Geometry check sheet. Reference: the model listing, model coordinates, mm. Face numbers are marked on the shaded views. A direction names the side the tool comes from. Coordinates: 2 decimals unless noted, no trailing zeros. Loops run counter-clockwise (first coordinate to the right, second up) from the corner with the lowest first, then second, coordinate; pieces in that order, holes last.
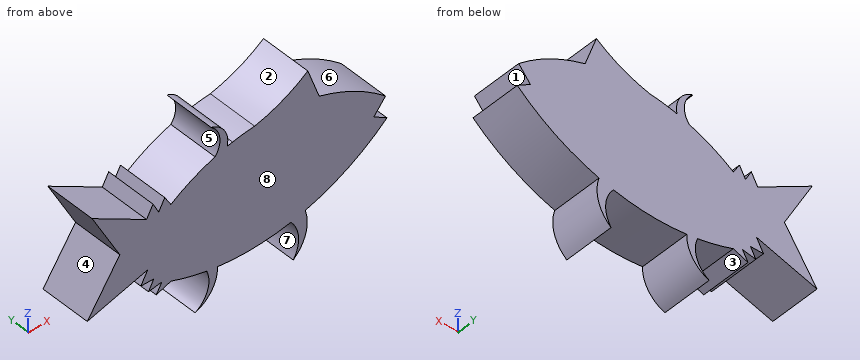
from build123d import *

# Parameters (mm, degrees)
F0_R     = 2.7728075116
F1_DEPTH = 25.4


with BuildPart() as f1:
    # F0 (on Front) → F1 (new body)
    with BuildSketch(Plane.XZ):
        with BuildLine():
            Line((-46.2063811719, 22.3736166954), (-73.4438300133, 37.6946814358))
            Line((-73.4438300133, 37.6946814358), (-59.5819167793, 12.4027663842))
            Line((-59.5819167793, 12.4027663842), (-75.8757442236, -11.4300008863))
            Line((-75.8757442236, -11.4300008863), (-45.6002619536, -2.5907051222))
            ThreePointArc((-45.6002619536, -2.5907051222), (-44.4025685397, -5.830070686), (-42.5679523522, -8.7561845276))
            ThreePointArc((-42.5679523522, -8.7561845276), (-40.7090131833, -10.7730955419), (-38.5467331667, -12.4607359072))
            ThreePointArc((-38.5467331667, -12.4607359072), (-37.5331692858, -13.0762341628), (-36.4787243307, -13.6187244207))
            ThreePointArc((-36.4787243307, -13.6187244207), (-35.218191008, -14.1097204461), (-33.9515178698, -14.5846525628))
            ThreePointArc((-33.9515178698, -14.5846525628), (-25.1236949217, -17.4009018565), (-16.0843420418, -19.4385027989))
            ThreePointArc((-16.0843420418, -19.4385027989), (-13.3899281297, -19.8880494602), (-10.6848629515, -20.2682874284))
            ThreePointArc((-10.6848629515, -20.2682874284), (7.7554033628, -21.0061419822), (26.0458368353, -18.5468952528))
            ThreePointArc((26.0458368353, -18.5468952528), (29.6524190677, -17.6722711402), (33.2263105994, -16.6724201227))
            ThreePointArc((33.2263105994, -16.6724201227), (54.9868951593, -7.4326700378), (74.1704591011, 6.3835123767))
            Line((74.1704591011, 6.3835123767), (67.6072314382, 10.4572335258))
            Line((67.6072314382, 10.4572335258), (73.4438300133, 17.5097864121))
            ThreePointArc((73.4438300133, 17.5097864121), (57.8267715443, 28.3623597624), (40.2292326492, 35.5732881621))
            ThreePointArc((40.2292326492, 35.5732881621), (24.2028822223, 38.5907293118), (7.8949533391, 38.5729912726))
            ThreePointArc((7.8949533391, 38.5729912726), (2.4157752889, 37.4790688574), (-3.1311035908, 36.8081045884))
            ThreePointArc((-3.1311035908, 36.8081045884), (-4.4740862067, 36.4927174845), (-5.8119143408, 36.1561358224))
            ThreePointArc((-5.8119143408, 36.1561358224), (-8.868524213, 35.3017374622), (-11.8920366653, 34.3367333588))
            ThreePointArc((-11.8920366653, 34.3367333588), (-23.3557486049, 29.5105094754), (-34.0166780636, 23.1031924486))
            Line((-34.0166780636, 23.1031924486), (-40.1115296178, 22.738404572))
            Line((-40.1115296178, 22.738404572), (-46.2063811719, 22.3736166954))
        make_face()
        with Locations((53.9885126054, 20.9144670516)):
            Circle(F0_R, mode=Mode.SUBTRACT)
        with BuildLine():
            ThreePointArc((34.5331951976, 51.0702133179), (21.8513167895, 43.4632987988), (7.8949533391, 38.5729912726))
            ThreePointArc((7.8949533391, 38.5729912726), (24.2028822223, 38.5907293118), (40.2292326492, 35.5732881621))
            Line((40.2292326492, 35.5732881621), (34.5331951976, 51.0702133179))
        make_face()
        with BuildLine():
            ThreePointArc((33.2263105994, -16.6724201227), (29.6524190677, -17.6722711402), (26.0458368353, -18.5468952528))
            ThreePointArc((26.0458368353, -18.5468952528), (29.9013197265, -27.9179314628), (27.237445116, -37.6946814358))
            ThreePointArc((27.237445116, -37.6946814358), (33.5352416657, -28.1246199246), (33.2263105994, -16.6724201227))
        make_face()
        with BuildLine():
            ThreePointArc((-10.6848629515, -20.2682874284), (-13.3899281297, -19.8880494602), (-16.0843420418, -19.4385027989))
            ThreePointArc((-16.0843420418, -19.4385027989), (-15.675284706, -29.1917075818), (-21.8872334808, -36.7219150066))
            ThreePointArc((-21.8872334808, -36.7219150066), (-13.5872618812, -30.3325564753), (-10.6848629515, -20.2682874284))
        make_face()
        with BuildLine():
            ThreePointArc((-13.8619150966, 49.8542524874), (-9.5317359626, 42.5201559061), (-11.8920366653, 34.3367333588))
            ThreePointArc((-11.8920366653, 34.3367333588), (-8.868524213, 35.3017374622), (-5.8119143408, 36.1561358224))
            ThreePointArc((-5.8119143408, 36.1561358224), (-7.128420184, 44.5969007804), (-13.8619150966, 49.8542524874))
        make_face()
        with Locations((53.9885126054, 20.9144670516)):
            Circle(F0_R)
        with BuildLine():
            ThreePointArc((-42.5679523522, -8.7561845276), (-44.4025685397, -5.830070686), (-45.6002619536, -2.5907051222))
            Line((-45.6002619536, -2.5907051222), (-49.0683440665, -8.7561845276))
            Line((-49.0683440665, -8.7561845276), (-42.5679523522, -8.7561845276))
        make_face()
        Polygon((-42.965512128, 28.13516175), (-46.2063811719, 22.3736166954), (-40.1115296178, 22.738404572), align=None)
        Polygon((-37.0758537513, 28.13516175), (-40.1115296178, 22.738404572), (-34.0166780636, 23.1031924486), align=None)
        with BuildLine():
            ThreePointArc((-38.5467331667, -12.4607359072), (-40.7090131833, -10.7730955419), (-42.5679523522, -8.7561845276))
            Line((-42.5679523522, -8.7561845276), (-45.233618468, -13.6187234893))
            Line((-45.233618468, -13.6187234893), (-38.5467331667, -12.4607359072))
        make_face()
        with BuildLine():
            ThreePointArc((-36.4787243307, -13.6187244207), (-37.5331692858, -13.0762341628), (-38.5467331667, -12.4607359072))
            Line((-38.5467331667, -12.4607359072), (-41.3425527513, -17.2665957361))
            Line((-41.3425527513, -17.2665957361), (-33.9515178698, -14.5846525628))
            ThreePointArc((-33.9515178698, -14.5846525628), (-35.218191008, -14.1097204461), (-36.4787243307, -13.6187244207))
        make_face()
        with BuildLine():
            ThreePointArc((7.8949533391, 38.5729912726), (2.3536609221, 37.8671258081), (-3.1311035908, 36.8081045884))
            ThreePointArc((-3.1311035908, 36.8081045884), (2.4157752889, 37.4790688574), (7.8949533391, 38.5729912726))
        make_face()
    extrude(amount=F1_DEPTH)


solid = f1.part
1) Mould release check, pull along Z, two halves, no side actions. Record for the marked faces 6, 7 and 8: +Z half, -Z half, draft (parallel to the pull), parting line (faces both ways), or undercut.
Data:
face 6: +Z half
face 7: undercut
face 8: draft
2) Section check C-C on z = 30. Record the cut outline in (x, y), and give its area (3 significant figures).
Data:
outline: (-69.23, -25.4) - (-59.76, -25.4) - (-59.76, 0) - (-69.23, 0) - close; (-22.38, -25.4) - (54.66, -25.4) - (54.66, 0) - (-22.38, 0) - close
area: 2,200 mm2
3) Material ranges on probe 1 along Z at (x, y) = (68, -3.25); probe 2 along Z at (x, y) = (-16, -21); probe 3 along X at (y, z) = (-10.75, 30.5), recorded low to high.
Data:
probe 1: z = 1.21 to 10.21, 10.93 to 21.88
probe 2: z = -33.15 to -30.06, -19.64 to 32.83
probe 3: x = -69.5 to -60.65, -21.34 to 53.63
4) Depth check by flat-ended pin: pin 1 (6 mm diameter, centred on x = -48, y = -3, fed in from +Z); pin 2 (1 mm diameter, centred on x = 55, z = -4.5, fed in from +Y); pin 3 (6 mm diameter, centred on y = -12, z = -24, fed in from -X); pin 4 (6 mm diameter, centred on x = -34, y = -8.5, fed in from +Z). Enter the tip coordinate at first touch or a pass-through.
Data:
pin 1: stops at z = 25.07
pin 2: stops at y = 0
pin 3: stops at x = -15.52
pin 4: stops at z = 28.01
5) Access from +Z, -Z, +X, -X, +Y, -Y to the whole of each face (thin tool, end or side, straight path). Record for the marked faces 1, 2, 3, 4 and 5.
Data:
face 1: +X, +Y, -Y
face 2: +Z, +Y, -Y
face 3: -Z, +Y, -Y
face 4: -X, +Y, -Y
face 5: +Y, -Y
6) Section check A-A on z = 44. Record the cut outline in (x, y).
Data:
outline: (-9.83, -25.4) - (-6.8, -25.4) - (-6.8, 0) - (-9.83, 0) - close; (22.97, -25.4) - (37.13, -25.4) - (37.13, 0) - (22.97, 0) - close
7) Section check D-D on x = 10. Record the cut outline in (y, z), and give its area (3 significant figures).
Data:
outline: (-25.4, -20.88) - (0, -20.88) - (0, 39.11) - (-25.4, 39.11) - close
area: 1,520 mm2
